Part model, mm, in its own coordinate system. Coordinates: 2 decimals unless noted, no trailing zeros. Loops run counter-clockwise (first coordinate to the right, second up) from the corner with the lowest first, then second, coordinate; pieces in that order, holes last. Notation, with made-up numbers: (-29.5, -19) - (25.5, -19) arc R17 cw to (25.5, 8) - close; hole circle Ø2 at (30.5, -13.5). An arc over 180 degrees is marked (long way). Use a Markdown table: item, result. Add a question column.
1) Probe probe 1 along Y at (x, z) = (0, 13.4); probe 2 along Z at (x, y) = (-2.5, -5); probe 3 along X at (y, z) = (-5.25, 16.5). List the from-to ranges inside material, lowest first. Write a range as [from, to].
2) Band-saw the part on B-B (z = 24). Give the cut face in (x, y), plus the area to 3 significant figures.
3) Drop flat-ended pins along their axis: P1, Ø8, axis at x = 3.5, y = -1.5, coming from the -Z side; P2, Ø1, axis at x = 0, y = -5.75, coming from the +Z side; P3, Ø1.4, axis at x = 0, y = 5.75, coming from the +Z side; P4, Ø1.5, axis at x = -5, z = 7.5, coming from the +Y side. Give the stop position or say it passes through.
4) Band-saw the part on A-A (y = 0). Give the cut face in (x, z), plus the area to 3 significant figures.
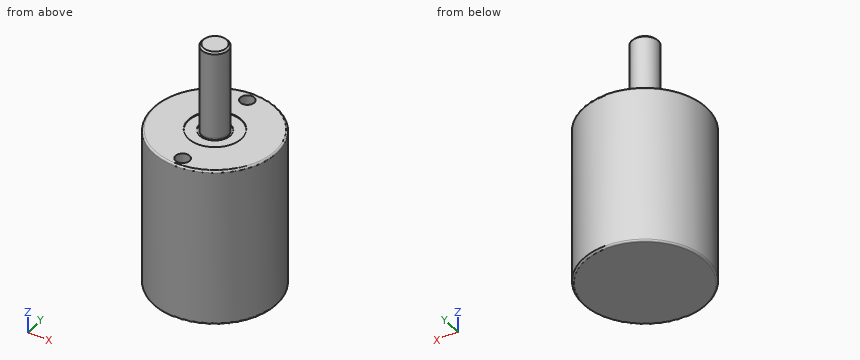
from build123d import *

# Parameters (mm, degrees)
SKETCH_1_R             = 7
EXTRUDE_1_DEPTH        = 18
FILLET_1_R             = 0.2
SKETCH_2_R             = 1.5
EXTRUDE_2_DEPTH        = 10
CHAMFER_1_SIZE         = 0.2
HOLE_WIZARD_M2_1_D     = 1.6
HOLE_WIZARD_M2_1_DEPTH = 6
HOLE_WIZARD_M2_1_TIP   = 0.480688495
SKETCH_6_R             = 1.75
SKETCH_6_R_2           = 1.5
CUT_EXTRUDE_1_DEPTH    = 0.2
SKETCH_7_R             = 3
SKETCH_7_R_2           = 1.75
CUT_EXTRUDE_2_DEPTH    = 0.1


with BuildPart() as part:
    # 草图1 → 凸台-拉伸1 (new body)
    with BuildSketch(Plane.XY):
        Circle(SKETCH_1_R)
    extrude(amount=EXTRUDE_1_DEPTH)

    # 圆角1
    fillet_1_edges = [part.edges().sort_by_distance(p)[0] for p in [
        (-7, 0, 0),
        (-7, 0, 18),
    ]]
    fillet(fillet_1_edges, radius=FILLET_1_R)

    # 草图2 → 凸台-拉伸2 (add)
    with BuildSketch(Plane.XY.offset(18)):
        Circle(SKETCH_2_R)
    extrude(amount=EXTRUDE_2_DEPTH)

    # 倒角1
    chamfer_1_edges = [part.edges().sort_by_distance(p)[0] for p in [
        (-1.5, 0, 28),
    ]]
    chamfer(chamfer_1_edges, length=CHAMFER_1_SIZE)

    # M2 螺纹孔1
    with Locations(Plane(origin=(0, 5.75, 18), x_dir=(1, 0, 0), z_dir=(0, 0, 1))):
        with Locations((0, 0), (0, -11.5)):
            Hole(HOLE_WIZARD_M2_1_D / 2, depth=HOLE_WIZARD_M2_1_DEPTH)
            with Locations((0, 0, -(HOLE_WIZARD_M2_1_DEPTH + HOLE_WIZARD_M2_1_TIP / 2))):  # 118° drill point
                Cone(0, HOLE_WIZARD_M2_1_D / 2, HOLE_WIZARD_M2_1_TIP, mode=Mode.SUBTRACT)

    # 草图6 → 切除-拉伸1 (cut)
    with BuildSketch(Plane.XY.offset(18)):
        Circle(SKETCH_6_R)
        Circle(SKETCH_6_R_2, mode=Mode.SUBTRACT)
    extrude(amount=-CUT_EXTRUDE_1_DEPTH, mode=Mode.SUBTRACT)

    # 草图7 → 切除-拉伸2 (cut)
    with BuildSketch(Plane.XY.offset(18)):
        Circle(SKETCH_7_R)
        Circle(SKETCH_7_R_2, mode=Mode.SUBTRACT)
    extrude(amount=-CUT_EXTRUDE_2_DEPTH, mode=Mode.SUBTRACT)


solid = part.part
Answer block:
| question | item | result |
|---|---|---|
| 1 | probe 1 | [-7, -6.55], [-4.95, 4.95], [6.55, 7] |
| 1 | probe 2 | [0, 18] |
| 1 | probe 3 | [-4.63, -0.62], [0.62, 4.63] |
| 2 | outline | circle Ø3 at (0, 0) |
| 2 | area | 7.07 mm2 |
| 3 | P1 | z = 0 |
| 3 | P2 | z = 11.82 |
| 3 | P3 | z = 11.94 |
| 3 | P4 | y = 5.56 |
| 4 | outline | (-7, 0.2) arc R0.2 ccw to (-6.8, 0) - (6.8, 0) arc R0.2 ccw to (7, 0.2) - (7, 17.8) arc R0.2 ccw to (6.8, 18) - (3, 18) - (3, 17.9) - (1.75, 17.9) - (1.75, 17.8) - (1.5, 17.8) - (1.5, 27.8) - (1.3, 28) - (-1.3, 28) - (-1.5, 27.8) - (-1.5, 17.8) - (-1.75, 17.8) - (-1.75, 17.9) - (-3, 17.9) - (-3, 18) - (-6.8, 18) arc R0.2 ccw to (-7, 17.8) - close |
| 4 | area | 282 mm2 |
